Input: part model. Units: mm. Frame: model coordinates. A direction names the side the tool comes from. Round coordinates to 2 decimals unless told otherwise and drop trailing zeros. Loops run counter-clockwise (first coordinate to the right, second up) from the corner with the lowest first, then second, coordinate; pieces in that order, holes last.
1) Ray query, line 1 along Y through (x, z) = (-4.6, 1); line 2 along Y through (x, z) = (4.4, 1.9); line 3 along Y through (x, z) = (-13.6, 2.25). Return the intervals inside material, ascending.
2) Draft query along Z for faces 1 (the face through (-21.067, 12.765, 10.605)), 2 (the face through (0, -37, 1.5)), 3 (the face through (22, -5.01, 11)). Return one class per face: pulls with the +Z half, pulls with the -Z half, needs draft (parallel to the pull), parting line crosses it, or undercut.
3) Access query for faces 4 (the face through (-22, 20.76, 11)), 5 (the face through (4, -37, 2)), 6 (the face through (22, -20.76, 11)), 7 (the face through (-8.06, -35, 9)). Directions: +Z, -Z, +X, -X, +Y, -Y. A direction counts if a zero-diameter tool reaches every point of the face in a straight line with its end or side. Return the directions, or none.
4) Section A-A, the plane y = -7.1. Return loops of the section in (x, z), and give its area (3 significant figures).
5) Section C-C, the plane z = 13. State how many separate pieces and enclosed holes the cut face has, and give its area (3 significant figures).
6) First-contact query: pin 1 (3 mm diameter, centred on x = 22, z = 11.5, fed in from +Y); pin 2 (6.5 mm diameter, centred on x = -4.6, y = -23.1, fed in from +Z); pin 3 (4 mm diameter, centred on x = -22, z = 12, fed in from -Y); pin 4 (0.6 mm diameter, centred on y = 36.5, z = 11.5, fed in from -X). Flat tips, straight axial feed; report the tip coordinate or a pass-through.
7) Section B-B, the plane x = 13.4. Return loops of the section in (y, z), and give its area (3 significant figures).
8) Section D-D, the plane y = -23.1. Return loops of the section in (x, z), and give its area (3 significant figures).
from build123d import *

# Parameters (mm, degrees)
CROQUIS1_W              = 50.8
CROQUIS1_H              = 76.2
SALIENTE_EXTRUIR1_DEPTH = 18
CROQUIS2_W              = 50.8
CROQUIS2_H              = 76.2
CROQUIS2_W_2            = 46.12
CROQUIS2_H_2            = 71.52
CROQUIS2_W_3            = 38.8
CROQUIS2_H_3            = 64.2
CORTAR_EXTRUIR1_DEPTH   = 15
CORTAR_EXTRUIR8_DEPTH   = 15
SALIENTE_EXTRUIR3_DEPTH = 41.5
CORTAR_EXTRUIR9_DEPTH   = 51.5
CORTAR_EXTRUIR10_DEPTH  = 51.5
SALIENTE_EXTRUIR4_DEPTH = 16
CORTAR_EXTRUIR11_DEPTH  = 16.5
REDONDEO3_R             = 2
REDONDEO4_R             = 1
CROQUIS15_W             = 48.12
CROQUIS15_H             = 10
CORTAR_EXTRUIR12_DEPTH  = 15
CROQUIS16_W             = 8
CROQUIS16_H             = 1.5
CORTAR_EXTRUIR13_DEPTH  = 2
CROQUIS17_R             = 4
CROQUIS17_R_2           = 3
CROQUIS17_R_3           = 3.105135185
CROQUIS17_R_4           = 3.001630679
CORTAR_EXTRUIR14_DEPTH  = 10


with BuildPart() as part:
    # Croquis1 → Saliente-Extruir1 (new body)
    with BuildSketch(Plane.XY):
        Rectangle(CROQUIS1_W, CROQUIS1_H)
    extrude(amount=SALIENTE_EXTRUIR1_DEPTH)

    # Croquis2 → Cortar-Extruir1 (cut)
    # profile 1 of 2: a face of its own
    with BuildSketch(Plane.XY.offset(18)):
        Rectangle(CROQUIS2_W, CROQUIS2_H)
        Rectangle(CROQUIS2_W_2, CROQUIS2_H_2, mode=Mode.SUBTRACT)
    # profile 2 of 2: a face of its own
    with BuildSketch(Plane.XY.offset(18)):
        Rectangle(CROQUIS2_W_3, CROQUIS2_H_3)
    extrude(amount=-CORTAR_EXTRUIR1_DEPTH, mode=Mode.SUBTRACT)

    # Croquis6 → Cortar-Extruir8 (cut)
    with BuildSketch(Plane.XY.offset(18)):
        Polygon((-23.06, 35.76), (-8.06, 35.76), (-8.06, 32.1), (-19.4, 32.1), (-19.4, 20.76), (-23.06, 20.76), align=None)
        Polygon((23.06, 35.76), (8.06, 35.76), (8.06, 32.1), (19.4, 32.1), (19.4, 20.76), (23.06, 20.76), align=None)
        Polygon((-23.06, -35.76), (-23.06, -20.76), (-19.4, -20.76), (-19.4, -32.1), (-8.06, -32.1), (-8.06, -35.76), align=None)
        Polygon((23.06, -35.76), (8.06, -35.76), (8.06, -32.1), (19.4, -32.1), (19.4, -20.76), (23.06, -20.76), align=None)
    extrude(amount=-CORTAR_EXTRUIR8_DEPTH, mode=Mode.SUBTRACT)

    # Croquis10 → Saliente-Extruir3 (add)
    with BuildSketch(Plane(origin=(0, -20.76, 0), x_dir=(-1, 0, 0), z_dir=(0, -1, 0))):
        Polygon((23.06, -18), (24.06, -18), (23.06, -3), align=None)
        Polygon((-23.06, -18), (-24.06, -18), (-23.06, -3), align=None)
    extrude(amount=-SALIENTE_EXTRUIR3_DEPTH)

    # Croquis11 → Cortar-Extruir9 (cut)
    with BuildSketch(Plane.XZ.offset(20.76)):
        Polygon((-19.4, 18), (-21.56, 18), (-20.56, 3), (-19.4, 3), align=None)
    extrude(amount=-CORTAR_EXTRUIR9_DEPTH, mode=Mode.SUBTRACT)

    # Croquis12 → Cortar-Extruir10 (cut)
    with BuildSketch(Plane.XZ.offset(20.76)):
        Polygon((19.4, 18), (19.4, 3), (20.56, 3), (21.56, 18), align=None)
    extrude(amount=-CORTAR_EXTRUIR10_DEPTH, mode=Mode.SUBTRACT)

    # Croquis13 → Saliente-Extruir4 (add)
    with BuildSketch(Plane(origin=(8.06, 0, 0), x_dir=(0, 0, -1), z_dir=(1, 0, 0))):
        Polygon((-18, -35.76), (-18, -37.76), (-3, -35.76), align=None)
        Polygon((-18, 35.76), (-18, 37.76), (-3, 35.76), align=None)
    extrude(amount=-SALIENTE_EXTRUIR4_DEPTH)

    # Croquis14 → Cortar-Extruir11 (cut)
    with BuildSketch(Plane(origin=(8.06, 0, 0), x_dir=(0, 0, -1), z_dir=(1, 0, 0))):
        Polygon((-3, -32.1), (-18, -32.1), (-18, -35.26), (-3, -33.26), align=None)
        Polygon((-18, 32.1), (-18, 35.26), (-3, 33.26), (-3, 32.1), align=None)
    extrude(amount=-CORTAR_EXTRUIR11_DEPTH, mode=Mode.SUBTRACT)

    # Redondeo3
    redondeo3_edges = [part.edges().sort_by_distance(p)[0] for p in [
        (-25.4, 38.1, 1.5),
        (25.4, 38.1, 1.5),
        (25.4, -38.1, 1.5),
        (-25.4, -38.1, 1.5),
    ]]
    fillet(redondeo3_edges, radius=REDONDEO3_R)

    # Redondeo4
    redondeo4_edges = [part.edges().sort_by_distance(p)[0] for p in [
        (0, 38.1, 0),
        (-25.4, 0, 0),
        (25.4, 0, 0),
        (0, -38.1, 0),
        (24.814213562, -37.514213562, 0),
        (-24.814213562, -37.514213562, 0),
        (-24.814213562, 37.514213562, 0),
        (24.814213562, 37.514213562, 0),
    ]]
    fillet(redondeo4_edges, radius=REDONDEO4_R)

    # Croquis15 → Cortar-Extruir12 (cut)
    with BuildSketch(Plane.XY.offset(18)):
        with Locations((0, -0.01)):
            Rectangle(CROQUIS15_W, CROQUIS15_H)
    extrude(amount=-CORTAR_EXTRUIR12_DEPTH, mode=Mode.SUBTRACT)

    # Croquis16 → Cortar-Extruir13 (cut)
    with BuildSketch(Plane.XZ.offset(38.1)):
        with Locations((0, 2.25)):
            Rectangle(CROQUIS16_W, CROQUIS16_H)
    extrude(amount=-CORTAR_EXTRUIR13_DEPTH, mode=Mode.SUBTRACT)

    # Croquis17 → Cortar-Extruir14 (cut)
    with BuildSketch(Plane.XY.offset(3)):
        with Locations((13.4, -23.1)):
            Circle(CROQUIS17_R)
        with Locations((13.4, -15.1)):
            Circle(CROQUIS17_R_2)
        with Locations((4.4, -23.1)):
            Circle(CROQUIS17_R)
        with Locations((-4.6, -23.1)):
            Circle(CROQUIS17_R)
        with Locations((-13.6, -23.1)):
            Circle(CROQUIS17_R)
        with Locations((4.4, -15.1)):
            Circle(CROQUIS17_R_2)
        with Locations((-4.6, -15.1)):
            Circle(CROQUIS17_R_2)
        with Locations((-13.6, -15.1)):
            Circle(CROQUIS17_R_2)
        with Locations((-4.6, -7.1)):
            Circle(CROQUIS17_R_3)
        with Locations((4.4, -7.1)):
            Circle(CROQUIS17_R_4)
    extrude(amount=-CORTAR_EXTRUIR14_DEPTH, mode=Mode.SUBTRACT)


solid = part.part
Final values:
1. line 1: y = -38.1 to -27.1, -19.1 to -18.1, -12.1 to -10.21, -3.99 to 38.1
1. line 2: y = -38.1 to -27.1, -19.1 to -18.1, -12.1 to -10.1, -4.1 to 38.1
1. line 3: y = -38.1 to -27.1, -19.1 to -18.1, -12.1 to 38.1
2. face 1: pulls with the +Z half
2. face 2: undercut
2. face 3: needs draft
3. face 4: +Z, +X, -X, +Y
3. face 5: -Y
3. face 6: +Z, +X, -X, -Y
3. face 7: +Z, -X, +Y, -Y
4. outline: (-25.4, 1) arc R1 ccw to (-24.4, 0) - (-7.71, 0) - (-7.71, 3) - (-20.56, 3) - (-21.56, 18) - (-24.06, 18) - (-23.06, 3) - (-25.4, 3) - close; (-1.49, 0) - (1.4, 0) - (1.4, 3) - (-1.49, 3) - close; (7.4, 0) - (24.4, 0) arc R1 ccw to (25.4, 1) - (25.4, 3) - (23.06, 3) - (24.06, 18) - (21.56, 18) - (20.56, 3) - (7.4, 3) - close
4. area: 190 mm2
5. separate pieces: 6
5. enclosed holes: 0
5. area: 238 mm2
6. pin 1: stops at y = 20.76
6. pin 2: passes through
6. pin 3: stops at y = -20.76
6. pin 4: stops at x = -7.94
7. outline: (-38.1, 1) arc R1 ccw to (-37.1, 0) - (-27.1, 0) - (-27.1, 3) - (-38.1, 3) - close; (-19.1, 0) - (-18.1, 0) - (-18.1, 3) - (-19.1, 3) - close; (-12.1, 0) - (37.1, 0) arc R1 ccw to (38.1, 1) - (38.1, 3) - (-12.1, 3) - close
7. area: 186 mm2
8. outline: (-25.4, 1) arc R1 ccw to (-24.4, 0) - (-17.6, 0) - (-17.6, 3) - (-25.4, 3) - close; (-9.6, 0) - (-8.6, 0) - (-8.6, 3) - (-9.6, 3) - close; (-0.6, 0) - (0.4, 0) - (0.4, 3) - (-0.6, 3) - close; (8.4, 0) - (9.4, 0) - (9.4, 3) - (8.4, 3) - close; (17.4, 0) - (24.4, 0) arc R1 ccw to (25.4, 1) - (25.4, 3) - (17.4, 3) - close
8. area: 56.0 mm2
